from build123d import *

# Parameters (mm, degrees)
F0_R     = 9.525
F0_R_2   = 7.366
F1_DEPTH = 19.05
F2_R     = 6.35
F3_DEPTH = 12.7
F4_W     = 7.6494621422
F4_H     = 6.35
F5_DEPTH = 12.7


# Not quite as in the source:
# - a fillet or chamfer that OpenCascade refuses, or shapes differently, is made with other operations: its cross-section is extruded or revolved along the edge and cut away or added


with BuildPart() as f1:
    # F0 (on Top) → F1 (new body, symmetric)
    with BuildSketch(Plane.XY):
        with Locations((-15.875, 0)):
            Circle(F0_R)
        with Locations((-15.875, 0)):
            Circle(F0_R_2, mode=Mode.SUBTRACT)
    extrude(amount=F1_DEPTH, both=True)



with BuildPart() as f1b:
    # F0 (on Top) → F1, piece 2 (new body, symmetric)
    with BuildSketch(Plane.XY):
        with Locations((15.875, 0)):
            Circle(F0_R)
        with Locations((15.875, 0)):
            Circle(F0_R_2, mode=Mode.SUBTRACT)
    extrude(amount=F1_DEPTH, both=True)


with BuildPart() as f1_1:
    add(f1.part)

    add(f1b.part)  # F3 merges F1b
    # F2 (on Top) → F3 (join, symmetric)
    with BuildSketch(Plane.XY):
        Circle(F2_R)
    extrude(amount=F3_DEPTH, both=True)

    # F4 (on Top) → F5 (join, symmetric)
    with BuildSketch(Plane.XY):
        with Locations((-3.8247310711, 3.175)):
            Rectangle(F4_W, F4_H)
        Polygon((7.4973143637, 0), (0, 0), (0, -6.35), (7.6071062533, -6.35), align=None)
    extrude(amount=F5_DEPTH, both=True)

    # F6: chamfer of 5.08 on 4 edges, made by hand

    # F6_s1 → F6_t2 (revolve, cut)
    with BuildSketch(Plane.XZ):
        Polygon((25.4, 13.97), (20.32, 19.05), (25.4, 19.05), align=None)
    revolve(axis=Axis((15.875, 0, 19.05), (0, 0, 1)), mode=Mode.SUBTRACT)

    # F6_s3 → F6_t4 (revolve, cut)
    with BuildSketch(Plane.XZ):
        Polygon((-6.35, 13.97), (-11.43, 19.05), (-6.35, 19.05), align=None)
    revolve(axis=Axis((-15.875, 0, 19.05), (0, 0, 1)), mode=Mode.SUBTRACT)

    # F6_s5 → F6_t6 (revolve, cut)
    with BuildSketch(Plane.XZ):
        Polygon((25.4, -13.97), (20.32, -19.05), (25.4, -19.05), align=None)
    revolve(axis=Axis((15.875, 0, -19.05), (0, 0, 1)), mode=Mode.SUBTRACT)

    # F6_s7 → F6_t8 (revolve, cut)
    with BuildSketch(Plane.XZ):
        Polygon((-6.35, -13.97), (-11.43, -19.05), (-6.35, -19.05), align=None)
    revolve(axis=Axis((-15.875, 0, -19.05), (0, 0, 1)), mode=Mode.SUBTRACT)


solid = f1_1.part
The listing builds one solid part. Answer for the finished solid, in the listing's coordinates (mm). Coordinates: 2 decimals unless noted, no trailing zeros. Loops run counter-clockwise (first coordinate to the right, second up) from the corner with the lowest first, then second, coordinate; pieces in that order, holes last.
1) Find the intervals of material crossed by L1, parallel to X at y = 5, z = 13; L2, parallel to Y at x = 0, z = 1; L3, parallel to Z at x = 1, y = -5.5, in increasing order.
2) Flat-ended cylindrical pins translate along their axes: pin 1 Ø4 at (x, y) = (3.5, -4.5) entering from +Z; pin 2 Ø6 at (x, z) = (3.5, 11) entering from +Y; pin 3 Ø4 at (x, z) = (-6, -11) entering from -Y; pin 4 Ø5 at (x, z) = (-14.5, -11.5) entering from +Y (3 decimals). Find the tip coordinate at first contact, or state that the pin passes through.
3) Find section C-C on x = 1. Write down the section's boundary in (y, z), then the cut area to 3 significant figures.
4) Find section A-A on z = 11.5. Write down the section's boundary in (x, y) (3 decimals), then the cut area to 3 significant figures.
5) Determine the mould class of faces 1 (the face through (-4, 6.35, 0)), 2 (the face through (4, -6.35, 0)), 3 (the face through (-8.85, 2.21, -0.23)), 4 (the face through (0, 0, -12.7)) for opening direction Y: pulls with the +Y half, pulls with the -Y half, needs draft (parallel to the pull), parting line crosses it, or undercut.
6) Find section B-B on y = -2.5. Give the number of separate pieces and of enclosed holes in the cut face, then the cut area to 3 significant figures.
Values:
1. L1: x = -23.98 to -21.28, -10.47 to -7.77, 7.77 to 10.47, 21.28 to 23.98
1. L2: y = -6.35 to 6.35
1. L3: z = -12.7 to 12.7
2. pin 1: stops at z = 12.7
2. pin 2: stops at y = 6.33
2. pin 3: stops at y = -5.36
2. pin 4: stops at y = 9.525
3. outline: (-6.35, -12.7) - (6.27, -12.7) - (6.27, 12.7) - (-6.35, 12.7) - close
3. area: 321 mm2
4. outline: (-7.649, 4.803) arc R9.525 ccw (long way) to (-6.35, 0) arc R6.35 ccw to (0, -6.35) - (7.607, -6.35) - (7.578, -4.679) arc R9.525 ccw (long way) to (6.35, 0) arc R6.35 ccw to (0, 6.35) - (-7.649, 6.35) - close; hole circle Ø14.732 at (-15.875, 0); hole circle Ø14.732 at (15.875, 0)
4. area: 381 mm2
5. face 1: pulls with the +Y half
5. face 2: pulls with the -Y half
5. face 3: undercut
5. face 4: needs draft
6. separate pieces: 4
6. enclosed holes: 0
6. area: 590 mm2
